The drawing under review shows one solid part. Ordinate dimensions are in mm from its lowest x, y, z. A direction names the side the tool comes from. Round coordinates to 2 decimals unless told otherwise and drop trailing zeros. Write each loop counter-clockwise with the first axis right and the second up, starting at its lowest first coordinate (ties: lowest second). Pieces come first, ordered by that corner, then holes. Notation, with made-up numbers: (26, 27) -> (80, 27) arc R17 ccw to (80, 56) -> close; hole circle Ø6 at (-39, 56.25). An arc over 180 degrees is marked (long way). Write item = value, one per line. Start each with the question number.
Item 1: Add section C-C, the plane z = 0.8. State the section outline as (x, y) points, then the cut area to 3 significant figures.
Item 2: To check wall thickness, follow L1, parallel to Y at x = 13, z = 2.1; L2, parallel to X at y = 6, z = 3.65; L3, parallel to Y at x = 25.5, z = 3.25. State the ranges of each line that lie inside material, in increasing order.
Item 3: Mouldability with a two-part tool opening along Y and no side actions: class the marked faces 3, 4, 5 and 6 as released by +Y, released by -Y, zero draft, split by the parting line, or undercut.
Item 4: Add section A-A, the plane y = 5. State the section outline as (x, z) points, then the cut area to 3 significant figures.
Item 5: Add section D-D, the plane y = 18. State the section outline as (x, z) points.
Item 6: Add section B-B, the plane x = 14.75. State the section outline as (y, z) points.
Item 7: Machinability: for the marked faces 1 and 2, which of the approach directions +Z, -Z, +X, -X, +Y, -Y give a long, thin tool a straight path to every point of the face, cutting with its end or side? Answer none if there is none.
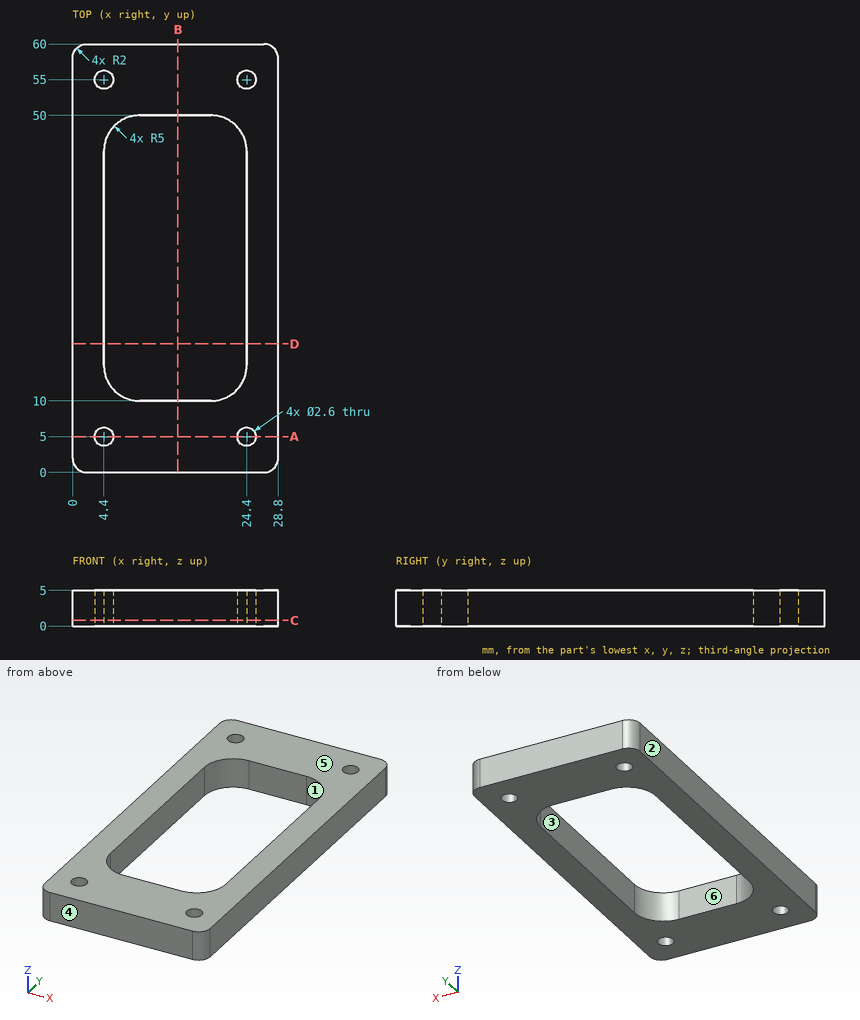
Result set:
q1.outline = (0, 2) arc R2 ccw to (2, 0) -> (26.8, 0) arc R2 ccw to (28.8, 2) -> (28.8, 58) arc R2 ccw to (26.8, 60) -> (2, 60) arc R2 ccw to (0, 58) -> close; hole circle Ø2.6 at (4.4, 5); hole circle Ø2.6 at (4.4, 55); hole (4.4, 15) arc R5 ccw to (9.4, 10) -> (19.4, 10) arc R5 ccw to (24.4, 15) -> (24.4, 45) arc R5 ccw to (19.4, 50) -> (9.4, 50) arc R5 ccw to (4.4, 45) -> close; hole circle Ø2.6 at (24.4, 5); hole circle Ø2.6 at (24.4, 55)
q1.area = 925 mm²
q2.L1 = 0 to 10, 50 to 60
q2.L2 = 0 to 3.57, 5.23 to 23.57, 25.23 to 28.8
q2.L3 = 0 to 4.31, 5.69 to 54.31, 55.69 to 60
q3.face_3 = undercut
q3.face_4 = released by -Y
q3.face_5 = zero draft
q3.face_6 = undercut
q4.outline = (0, 0) -> (3.1, 0) -> (3.1, 5) -> (0, 5) -> close; (5.7, 0) -> (23.1, 0) -> (23.1, 5) -> (5.7, 5) -> close; (25.7, 0) -> (28.8, 0) -> (28.8, 5) -> (25.7, 5) -> close
q4.area = 118 mm²
q5.outline = (0, 0) -> (4.4, 0) -> (4.4, 5) -> (0, 5) -> close; (24.4, 0) -> (28.8, 0) -> (28.8, 5) -> (24.4, 5) -> close
q6.outline = (0, 0) -> (10, 0) -> (10, 5) -> (0, 5) -> close; (50, 0) -> (60, 0) -> (60, 5) -> (50, 5) -> close
q7.face_1 = +Z, -Z
q7.face_2 = +Z, -Z, -X, +Y, -Y
